Autodesk Inventor part; units mm, degrees
ref_plane "YZ Plane" through (0, 0, 0) normal (1, 0, 0) x (0, 1, 0)
ref_plane "XZ Plane" through (0, 0, 0) normal (0, 1, 0) x (-1, 0, 0)
ref_plane "XY Plane" through (0, 0, 0) normal (0, 0, 1) x (1, 0, 0)
sketch "Sketch1" plane through (0, 0, 0) normal (0, 0, 1) x (1, 0, 0)
  circle A0 centre (17.6777, -17.6777) radius 3
  circle A1 centre (-17.6777, -17.6777) radius 3
  circle A2 centre (-17.6777, 17.6777) radius 3
  circle A3 centre (17.6777, 17.6777) radius 3
  circle A4 centre (-11.1369, -11.1369) radius 2.5
  circle A5 centre (11.1369, -11.1369) radius 2.5
  circle A6 centre (-11.1369, 11.1369) radius 2.5
  circle A7 centre (11.1369, 11.1369) radius 2.5
  arc A8 (-6.4273, -6.3) -> (-6.4273, 6.3) centre (0, 0) ccw
  arc A9 (-31.8835, -6.3) -> (-31.8835, 6.3) centre (0, 0) ccw
  circle A10 centre (0, 0) radius 32.5
  circle A11 centre (0, 0) radius 9
  line L0 (22.4721, 110) -> (-22.4721, 110)
  line L1 (-27.4721, 105) -> (-27.4721, 90)
  line L2 (-23.0608, 85.5886) -> (-23.0608, 31.884)
  line L3 (23.0603, 31.884) -> (23.0603, 85.5881)
  line L4 (27.4721, 90) -> (27.4721, 105)
  circle A12 centre (22.5, 100) radius 1.5
  circle A13 centre (-22.5, 100) radius 1.5
  circle A14 centre (11.1369, -11.1369) radius 2.5
  circle A15 centre (11.1369, 11.1369) radius 2.5
  circle A16 centre (-11.1369, 11.1369) radius 2.5
  circle A17 centre (-11.1369, -11.1369) radius 2.5
  line L5 (27.4721, 105) -> (27.4721, 110)
  line L6 (27.4721, 110) -> (-27.4721, 110)
  line L7 (-27.4721, 110) -> (-27.4721, 105)
  line L8 (27.4721, 90) -> (27.4721, 85.5881)
  line L9 (27.4721, 85.5881) -> (-27.4721, 85.5881)
  line L10 (-27.4721, 85.5881) -> (-27.4721, 90)
  line L11 (-23.0608, 31.884) -> (-23.0608, 22.9009)
  line L12 (23.0603, 31.884) -> (23.0603, 22.9014)
  point P0 (-31.8835, 6.3)
  point P1 (-23.0608, 85.5881)
  point P2 (-6.4273, 6.3)
extrude "Extrusion1" add sketch "Sketch1" along normal blind 5
fillet "Fillet1" radius 5 6 edges at (-27.4721, 110, 2.5) (27.4721, 110, 2.5) (-27.4721, 85.5881, 2.5) (-23.0608, 85.5881, 2.5) (27.4721, 85.5881, 2.5) (23.0603, 85.5881, 2.5)
sketch "Sketch2" plane through (0, 0, 5) normal (0, 0, 1) x (1, 0, 0)
  circle A0 centre (-22.5, 100) radius 1.5
  arc A1 (9, 70) -> (-9, 70) centre (0, 70) ccw
  line L0 (-9, 70) -> (-9, 50)
  line L1 (9, 70) -> (9, 50)
  line L2 (0, 40) -> (0, 50)
  arc A2 (-9, 50) -> (9, 50) centre (0, 50) ccw
  point P0 (0, 0)
  dimension "d9" = 18
  dimension "d12" = 10
  dimension "d13" = 18
extrude "Extrusion2" cut sketch "Sketch2" against normal blind 10 contours L1 A2 L0 A1
sketch "Sketch3" plane through (0, 0, 5) normal (0, 0, 1) x (1, 0, 0)
  circle A0 centre (-22.5, 100) radius 1.5
  circle A1 centre (-22.5, 100) radius 1.55
  circle A2 centre (22.5, 100) radius 1.5
  circle A3 centre (22.5, 100) radius 1.55
  circle A4 centre (-17.6777, 17.6777) radius 3
  circle A5 centre (-17.6777, 17.6777) radius 3.05
  circle A6 centre (17.6777, 17.6777) radius 3
  circle A7 centre (17.6777, 17.6777) radius 3.05
  circle A8 centre (11.1369, 11.1369) radius 2.5
  circle A9 centre (11.1369, 11.1369) radius 2.55
  circle A10 centre (-11.1369, 11.1369) radius 2.5
  circle A11 centre (-11.1369, 11.1369) radius 2.55
  circle A12 centre (-11.1369, -11.1369) radius 2.5
  circle A13 centre (-11.1369, -11.1369) radius 2.55
  circle A14 centre (11.1369, -11.1369) radius 2.5
  circle A15 centre (11.1369, -11.1369) radius 2.55
  circle A16 centre (-17.6777, -17.6777) radius 3
  circle A17 centre (-17.6777, -17.6777) radius 3.05
  circle A18 centre (17.6777, -17.6777) radius 3
  circle A19 centre (17.6777, -17.6777) radius 3.05
  point P0 (0, 0)
  dimension "d14" = 3.1
  dimension "d15" = 3.1
  dimension "d16" = 6.1
  dimension "d17" = 6.1
  dimension "d18" = 5.1
  dimension "d19" = 5.1
  dimension "d20" = 5.1
  dimension "d21" = 5.1
  dimension "d22" = 6.1
  dimension "d23" = 6.1
extrude "Extrusion3" cut sketch "Sketch3" against normal blind 10 contours A0 | A1 | A2 | A3 | A4 | A5 | A6 | A7 | A8 | A9 | A10 | A11 | A12 | A13 | A14 | A15 | A16 | A17 | A18 | A19
properties part number "Part2_Camera"
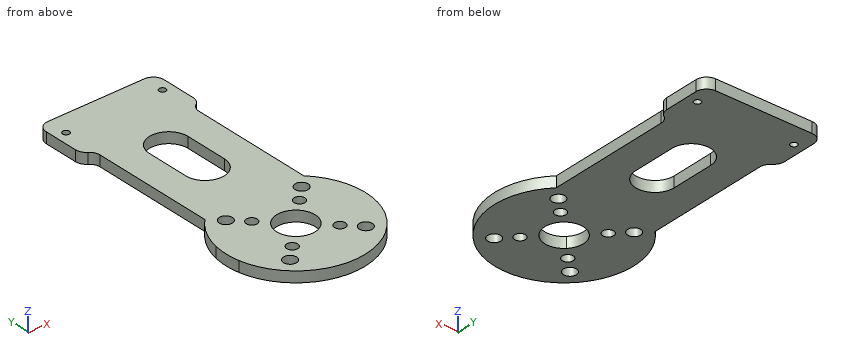
Design review of the part built by this model. Coordinates are the model's own, in mm. Coordinates: 2 decimals unless noted, no trailing zeros. Order: outer loops, then holes, each group sorted by start corner. A loop starts at its lowest first (then second) coordinate and runs counter-clockwise, first axis right, second up.
Item 1: Take a section at D-D, the plane z = 3.1. Count the separate pieces of the cut face and the enclosed holes in it, then the cut area to 3 significant figures.
Item 2: Take a section at C-C, the plane y = 0. Write out the cut boundary in (x, z), then the cut area to 3 significant figures.
Item 3: Take a section at B-B, the plane x = 0. Write out the cut boundary in (y, z), then the cut area to 4 significant figures.
Item 4: For pin 1 Ø2.5 at (y, z) = (50, 1.5) entering from -X; pin 2 Ø1 at (y, z) = (74.5, 0.5) entering from +X; pin 3 Ø1 at (x, z) = (-4, 2) entering from -Y, all flat-tipped, find the tip position at first contact; note any pin that passes through.
Item 5: Take a section at A-A, the plane y = 100. Write out the cut boundary in (x, z), then the cut area to 3 significant figures.
Item 6: For line 1 (Y direction, x = 11, z = 3.95); line 2 (X direction, y = -10, z = 1.4); line 3 (X direction, y = 70.5, z = 3.25), list the stretches that pass through material, from the lowest coordinate up.
The answers:
1. separate pieces: 1
1. enclosed holes: 12
1. area: 6,160 mm2
2. outline: (-32.5, 0) - (-9, 0) - (-9, 5) - (-32.5, 5) - close; (9, 0) - (32.5, 0) - (32.5, 5) - (9, 5) - close
2. area: 235 mm2
3. outline: (-32.5, 0) - (-9, 0) - (-9, 5) - (-32.5, 5) - close; (9, 0) - (41, 0) - (41, 5) - (9, 5) - close; (79, 0) - (110, 0) - (110, 5) - (79, 5) - close
3. area: 432.5 mm2
4. pin 1: stops at x = -23.06
4. pin 2: stops at x = 23.06
4. pin 3: stops at y = -32.31
5. outline: (-27.47, 0) - (-24.05, 0) - (-24.05, 5) - (-27.47, 5) - close; (-20.95, 0) - (20.95, 0) - (20.95, 5) - (-20.95, 5) - close; (24.05, 0) - (27.47, 0) - (27.47, 5) - (24.05, 5) - close
5. area: 244 mm2
6. line 1: y = -30.58 to -13.68, -8.59 to 8.59, 13.68 to 110
6. line 2: x = -30.92 to -13.42, -8.85 to 8.85, 13.42 to 30.92
6. line 3: x = -23.06 to -8.99, 8.99 to 23.06
